```python
from build123d import *

# Parameters (mm, degrees)
CROQUIS1_R              = 4.95
CROQUIS1_R_2            = 3.175
SALIENTE_EXTRUIR1_DEPTH = 5
CORTAR_EXTRUIR1_DEPTH   = 66.924198895


with BuildPart() as part:
    # Croquis1 → Saliente-Extruir1 (new body)
    with BuildSketch(Plane.XY):
        with BuildLine():
            Line((13, 0), (-13, 0))
            ThreePointArc((-13, 0), (-19.544656296, 4.709966775), (-24.061489507, 11.389377737))
            ThreePointArc((-24.061489507, 11.389377737), (-30, 21.95), (-35.938510493, 11.389377737))
            ThreePointArc((-35.938510493, 11.389377737), (-36.984260452, 5.34343649), (-40, 0))
            Line((-40, 0), (-55, 0))
            Line((-55, 0), (-55, -24))
            Line((-55, -24), (-25, -24))
            Line((-25, -24), (-25, -36))
            Line((-25, -36), (25, -36))
            Line((25, -36), (25, -24))
            Line((25, -24), (55, -24))
            Line((55, -24), (55, 0))
            Line((55, 0), (40, 0))
            ThreePointArc((40, 0), (36.984260452, 5.34343649), (35.938510493, 11.389377737))
            ThreePointArc((35.938510493, 11.389377737), (30, 21.95), (24.061489507, 11.389377737))
            ThreePointArc((24.061489507, 11.389377737), (19.544656296, 4.709966775), (13, 0))
        make_face()
        with Locations((-30, 15)):
            Circle(CROQUIS1_R, mode=Mode.SUBTRACT)
        with Locations((-37.5, -12)):
            Circle(CROQUIS1_R_2, mode=Mode.SUBTRACT)
        with Locations((0, -30)):
            Circle(CROQUIS1_R_2, mode=Mode.SUBTRACT)
        with Locations(Location((30, 15, 0), (0, 0, 180))):
            Circle(CROQUIS1_R, mode=Mode.SUBTRACT)
        with Locations(Location((37.5, -12, 0), (0, 0, 180))):
            Circle(CROQUIS1_R_2, mode=Mode.SUBTRACT)
        with Locations((-15, -30)):
            Circle(CROQUIS1_R_2, mode=Mode.SUBTRACT)
        with Locations(Location((15, -30, 0), (0, 0, 180))):
            Circle(CROQUIS1_R_2, mode=Mode.SUBTRACT)
    extrude(amount=SALIENTE_EXTRUIR1_DEPTH)

    # Croquis2 → Cortar-Extruir1 (cut, through all)
    with BuildSketch(Plane.XY):
        with BuildLine():
            Line((-30, 16.7), (-36.738879729, 16.7))
            ThreePointArc((-36.738879729, 16.7), (-36.95, 15), (-36.738879729, 13.3))
            Line((-36.738879729, 13.3), (-30, 13.3))
            Line((-30, 13.3), (-30, 16.7))
        make_face()
        with BuildLine():
            Line((30, 16.7), (30, 13.3))
            Line((30, 13.3), (36.738879729, 13.3))
            ThreePointArc((36.738879729, 13.3), (36.95, 15), (36.738879729, 16.7))
            Line((36.738879729, 16.7), (30, 16.7))
        make_face()
    extrude(amount=CORTAR_EXTRUIR1_DEPTH, mode=Mode.SUBTRACT)


solid = part.part
```
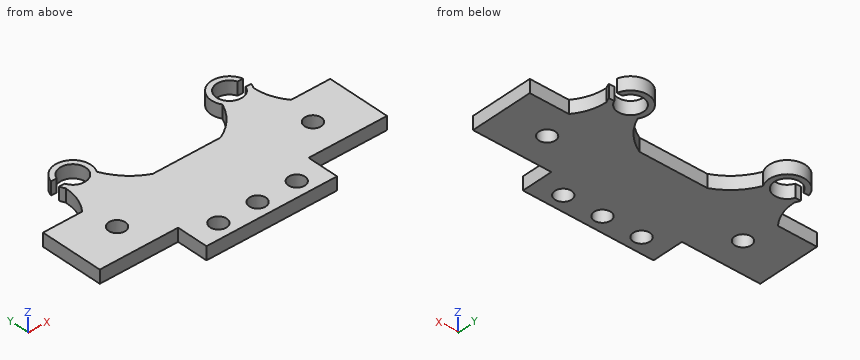
Input: part model. Units: mm. Frame: model coordinates. Coordinates: 2 decimals unless noted, no trailing zeros. Loops run counter-clockwise (first coordinate to the right, second up) from the corner with the lowest first, then second, coordinate; pieces in that order, holes last. Notation, with made-up numbers: (4.5, -14.5) -> (35.5, -14.5) arc R10 cw to (35.5, -2.5) -> close; hole circle Ø10 at (-32, 37.25). An arc over 180 degrees is marked (long way). Use a Markdown table: item, result.
1) Cut plane B-B (x = 0). Return the cut outline in (y, z) (3 decimals), then the cut area to 3 significant figures.
Results found:
| item | result |
|---|---|
| outline | (-36, 0) -> (-33.175, 0) -> (-33.175, 5) -> (-36, 5) -> close; (-26.825, 0) -> (0, 0) -> (0, 5) -> (-26.825, 5) -> close |
| area | 148 mm2 |
2) Material intervals for line 1 along Y through (x, z) = (-30, 1.75); line 2 along X through (y, z) = (-27.5, 3.2); line 3 along Y through (x, z) = (0, 2.65) (3 decimals), sorted ascending. Write a range as from..to.
Results found:
| item | result |
|---|---|
| line 1 | y = -24..10.05, 19.95..21.95 |
| line 2 | x = -25..-16.96, -13.04..-1.96, 1.96..13.04, 16.96..25 |
| line 3 | y = -36..-33.175, -26.825..0 |
3) Contact query for flat-ended pins moving along their axis: pin 1 (0.6 mm diameter, centred on x = -35.5, z = 3.5, fed in from -Y); pin 2 (1 mm diameter, centred on x = -35.5, z = 2, fed in from +Y); pin 3 (1.5 mm diameter, centred on x = -3.5, z = 2, fed in from +Y). Output: stop coordinate, or through.
Results found:
| item | result |
|---|---|
| pin 1 | stops at y = -24 |
| pin 2 | stops at y = 19.83 |
| pin 3 | stops at y = 0 |
4) Cut plane A-A (y = -12). Return the cut outline in (x, z) (3 decimals).
Results found:
| item | result |
|---|---|
| outline | (-55, 0) -> (-40.675, 0) -> (-40.675, 5) -> (-55, 5) -> close; (-34.325, 0) -> (34.325, 0) -> (34.325, 5) -> (-34.325, 5) -> close; (40.675, 0) -> (55, 0) -> (55, 5) -> (40.675, 5) -> close |
5) Cut plane C-C (y = -30). Return the cut outline in (x, z) (3 decimals).
Results found:
| item | result |
|---|---|
| outline | (-25, 0) -> (-18.175, 0) -> (-18.175, 5) -> (-25, 5) -> close; (-11.825, 0) -> (-3.175, 0) -> (-3.175, 5) -> (-11.825, 5) -> close; (3.175, 0) -> (11.825, 0) -> (11.825, 5) -> (3.175, 5) -> close; (18.175, 0) -> (25, 0) -> (25, 5) -> (18.175, 5) -> close |
6) Cut plane D-D (z = 2.3). Give the number of separate pieces and of enclosed holes in the cut face, then the cut area to 3 significant figures.
Results found:
| item | result |
|---|---|
| separate pieces | 1 |
| enclosed holes | 5 |
| area | 3,560 mm2 |
